Source: three-view drawing plus pictorial views. Frame: mm from the lowest corner of the part. A direction names the side the tool comes from. Give positions to 0.01 mm unless a question says otherwise; leave off trailing zeros. Order: outer loops, then holes, each group sorted by start corner. A loop starts at its lowest first (then second) coordinate and runs counter-clockwise, first axis right, second up.
1) Access query for the marked faces 1, 2 and 3. Directions: +Z, -Z, +X, -X, +Y, -Y. A direction counts if a zero-diameter tool reaches every point of the face in a straight line with its end or side. Return the directions, or none.
2) Draft query along X for the marked faces 4, 5 and 6. Return one class per face: released by +X, released by -X, zero draft, split by the parting line, or undercut.
3) Material intervals for line 1 (X direction, y = 48.5, z = 2.75); line 2 (Y direction, x = 61, z = 7.75); line 3 (X direction, y = 120, z = 1.25), sorted ascending.
4) Section C-C, the plane y = 44.5. Return loops of the section in (x, z).
5) First-contact query: P1, Ø5, axis at x = 59, z = 4.5, coming from the -Y side; P2, Ø3, axis at x = 15, z = 4.5, coming from the +Y side; P3, Ø6.5, axis at y = 112.5, z = 9, coming from the -X side; P4, Ø5, axis at y = 17, z = 10, coming from the -X side. Flat tips, straight axial feed; report the tip coordinate or a pass-through.
6) Section B-B, the plane z = 4.75. Return loops of the section in (x, y), plus the area to 3 significant figures.
7) Section A-A, the plane x = 40. Return loops of the section in (y, z), plus the area to 3 significant figures.
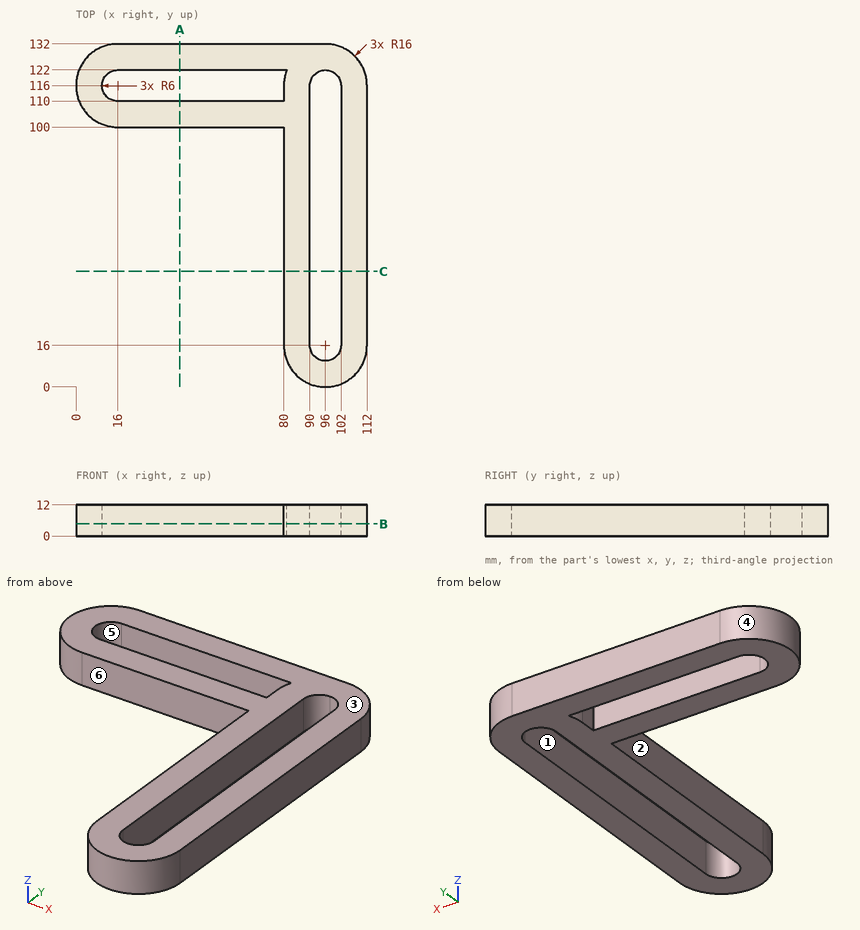
From the geometry:
1. face 1: +Z, -Z
1. face 2: +Z, -Z, -X, -Y
1. face 3: +Z, +X, -X, +Y, -Y
2. face 4: released by -X
2. face 5: undercut
2. face 6: zero draft
3. line 1: x = 80 to 90, 102 to 112
3. line 2: y = 100 to 110, 122 to 132
3. line 3: x = 0.51 to 11.53, 80.51 to 91.53, 100.47 to 111.49
4. outline: (80, 0) - (90, 0) - (90, 12) - (80, 12) - close; (102, 0) - (112, 0) - (112, 12) - (102, 12) - close
5. P1: stops at y = 100
5. P2: stops at y = 132
5. P3: stops at x = 0
5. P4: stops at x = 80
6. outline: (16, 100) - (80, 100) - (80, 16) arc R16 ccw to (112, 16) - (112, 116) arc R16 ccw to (96, 132) - (16, 132) arc R16 ccw to start; hole (16, 110) - (80, 110) - (80, 116) arc R16 cw to (81.17, 122) - (16, 122) arc R6 ccw to start; hole (90, 16) arc R6 ccw to (102, 16) - (102, 116) arc R6 ccw to (90, 116) - close
6. area: 4,370 mm2
7. outline: (100, 0) - (110, 0) - (110, 12) - (100, 12) - close; (122, 0) - (132, 0) - (132, 12) - (122, 12) - close
7. area: 240 mm2
